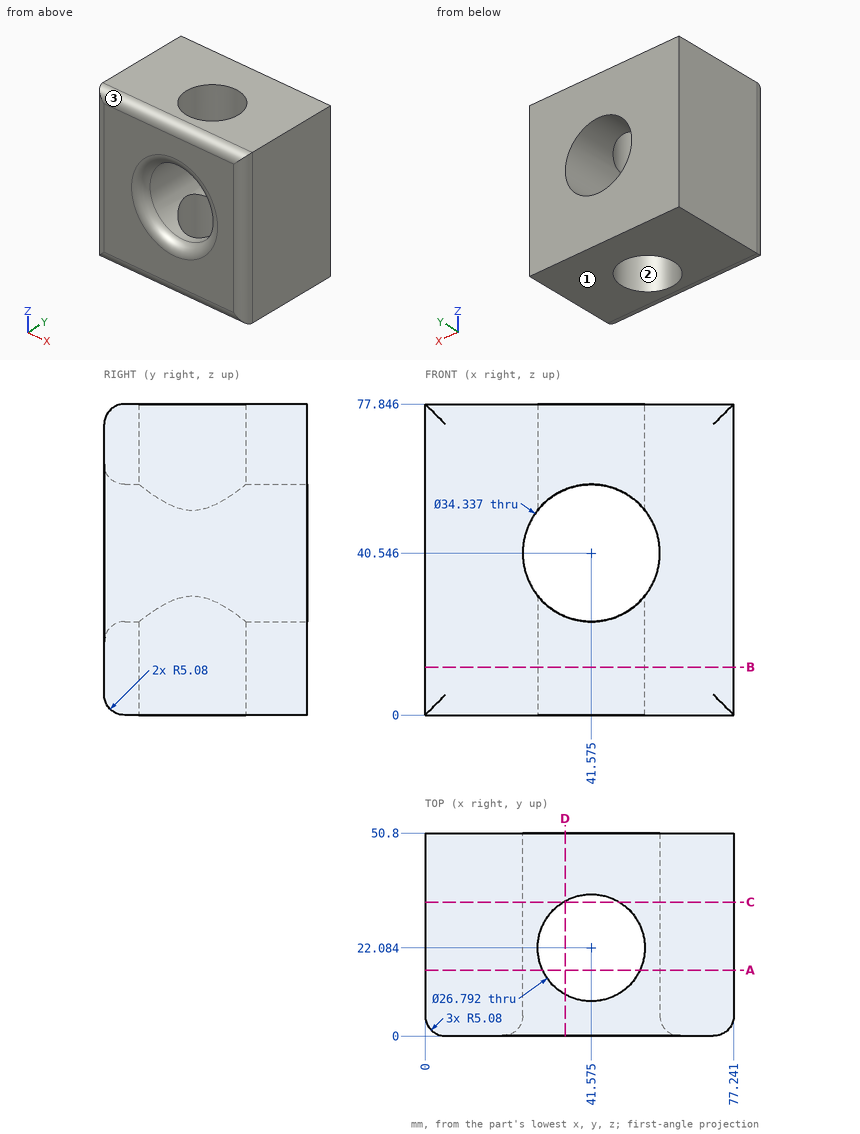
Print and shaded views of the part. All mm, measured from the part's lowest x, y and z. Round coordinates to 2 decimals unless told otherwise and drop trailing zeros. Write each loop counter-clockwise with the first axis right and the second up, starting at its lowest first coordinate (ties: lowest second). Pieces come first, ordered by that corner, then holes. Notation, with made-up numbers: (52, 46.5) -> (98, 46.5) arc R21 cw to (98, 67.5) -> close; hole circle Ø2 at (36.5, 24.25). An arc over 180 degrees is marked (long way). Write item = value, one per line.
(1) Probe L1, parallel to X at y = 25, z = 40 (1 decimal); L2, parallel to Y at x = 52.5, z = 67 (1 decimal); L3, parallel to Z at x = 33, y = 39 (1 decimal). List the from-to ranges inside material, lowest first.
Answer:
L1 = 0 to 24.4, 58.7 to 77.2
L2 = 0 to 14.3, 29.8 to 50.8
L3 = 0 to 25.7, 55.4 to 77.8
(2) Two-plate mould, pull along Y, no slides. Class the marked faces 1, 2 and 3: pulls with the +Y half, pulls with the -Y half, needs draft (parallel to the pull), parting line crosses it, or undercut.
Answer:
face_1 = needs draft
face_2 = undercut
face_3 = pulls with the -Y half
(3) Band-saw the part on C-C (y = 33.5). Give the cut face in (x, z) (1 decimal).
Answer:
outline = (0, 0) -> (34.6, 0) -> (34.6, 24.9) arc R17.2 cw to (34.6, 56.2) -> (34.6, 77.8) -> (0, 77.8) -> close; (48.6, 0) -> (77.2, 0) -> (77.2, 77.8) -> (48.6, 77.8) -> (48.6, 56.2) arc R17.2 cw to (48.6, 24.9) -> close
(4) Band-saw the part on B-B (z = 12). Give the cut face in (x, y) (1 decimal).
Answer:
outline = (0, 5.1) arc R5.1 ccw to (5.1, 0) -> (72.2, 0) arc R5.1 ccw to (77.2, 5.1) -> (77.2, 50.8) -> (0, 50.8) -> close; hole circle Ø26.8 at (41.6, 22.1)
(5) Band-saw the part on A-A (y = 16.5). Give the cut face in (x, z) (1 decimal).
Answer:
outline = (0, 0) -> (29.4, 0) -> (29.4, 28.4) arc R17.2 cw to (29.4, 52.6) -> (29.4, 77.8) -> (0, 77.8) -> close; (53.8, 0) -> (77.2, 0) -> (77.2, 77.8) -> (53.8, 77.8) -> (53.8, 52.6) arc R17.2 cw to (53.8, 28.4) -> close
(6) Band-saw the part on D-D (x = 35). State how many separate pieces and enclosed holes the cut face has, then the cut area to 3 significant figures.
Answer:
separate_pieces = 4
enclosed_holes = 0
area = 1,240 mm2
